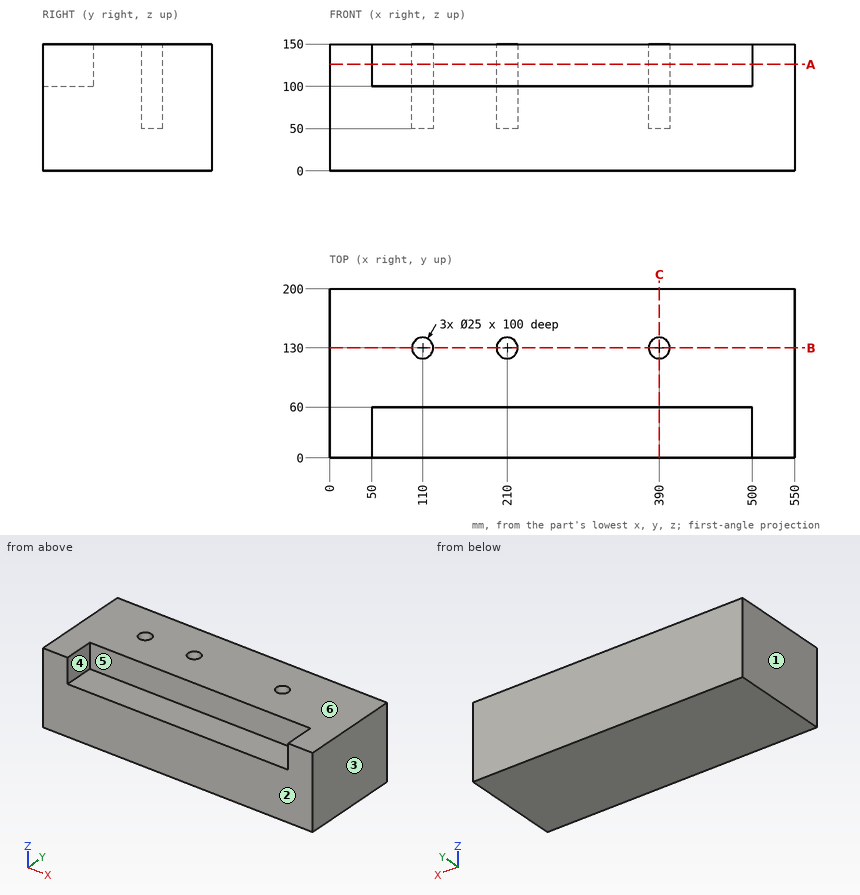
Check sheet for the drawn part. Datum: minimum x, y, z corner. Units: mm. A direction names the side the tool comes from. Give positions to 0.01 mm unless a question says otherwise; leave off trailing zeros. Order: outer loops, then holes, each group sorted by start corner. A loop starts at its lowest first (then second) coordinate and runs counter-clockwise, first axis right, second up. Notation, with made-up numbers: (-1, 1) - (47, 1) arc R28 cw to (47, 37) - close; hole circle Ø8 at (-14, -6). An arc over 180 degrees is marked (long way). Answer in a Markdown table with one row per item. Add a question column.
Q1. Tool access check on the marked faces 5 and 6. Record the directions out of +Z, -Z, +X, -X, +Y, -Y that give a thin tool (end or side, any length) a straight path to the whole face; none if there is none.
Q2. Mould release check, pull along X, two halves, no side actions. Record for the marked faces 1, 2, 3 and 4: pulls with the +X half, pulls with the -X half, needs draft (parallel to the pull), parting line crosses it, or undercut.
Q3. Cross-section at A-A, the plane z = 126. Enter the section's corners in (x, y), then the cut area to 3 significant figures.
Q4. Material ranges on probe 1 along X at (y, z) = (42, 107.5); probe 2 along Y at (x, z) = (210, 102); probe 3 along Y at (x, z) = (110, 77.5), recorded low to high. Write a range as from..to.
Q5. Cross-section at C-C, the plane x = 390. Enter the section's corners in (y, z), then the cut area to 3 significant figures.
Q6. Gauge pin test, flat end, axial feed: pin 1 (12.5 mm diameter, centred on x = 395, y = 133.5, fed in from +Z). Record the tip position at first contact, or that the pin passes through.
Q7. Cross-section at B-B, the plane y = 130. Enter the section's corners in (x, z).
Check values:
| question | item | result |
|---|---|---|
| 1 | face 5 | +Z, -Y |
| 1 | face 6 | +Z, +X, -X, +Y, -Y |
| 2 | face 1 | pulls with the -X half |
| 2 | face 2 | needs draft |
| 2 | face 3 | pulls with the +X half |
| 2 | face 4 | undercut |
| 3 | outline | (0, 0) - (50, 0) - (50, 60) - (500, 60) - (500, 0) - (550, 0) - (550, 200) - (0, 200) - close; hole circle Ø25 at (110, 130); hole circle Ø25 at (210, 130); hole circle Ø25 at (390, 130) |
| 3 | area | 81,500 mm^2 |
| 4 | probe 1 | x = 0..50, 500..550 |
| 4 | probe 2 | y = 60..117.5, 142.5..200 |
| 4 | probe 3 | y = 0..117.5, 142.5..200 |
| 5 | outline | (0, 0) - (200, 0) - (200, 150) - (142.5, 150) - (142.5, 50) - (117.5, 50) - (117.5, 150) - (60, 150) - (60, 100) - (0, 100) - close |
| 5 | area | 24,500 mm^2 |
| 6 | pin 1 | stops at z = 50 |
| 7 | outline | (0, 0) - (550, 0) - (550, 150) - (402.5, 150) - (402.5, 50) - (377.5, 50) - (377.5, 150) - (222.5, 150) - (222.5, 50) - (197.5, 50) - (197.5, 150) - (122.5, 150) - (122.5, 50) - (97.5, 50) - (97.5, 150) - (0, 150) - close |
